Work out the finished part from the listing and answer in its coordinate system (mm). Coordinates: 2 decimals unless noted, no trailing zeros. Order: outer loops, then holes, each group sorted by start corner. A loop starts at its lowest first (then second) coordinate and runs counter-clockwise, first axis right, second up. Notation, with made-up numbers: (54, -4.75) -> (92, -4.75) arc R20 cw to (92, 29.25) -> close; hole circle Ø5 at (16.25, 82). An arc over 180 degrees is marked (long way). Use one line per item in the form item = value.
from build123d import *

# Parameters (mm, degrees)
F1_DEPTH      = 25.4
F1_DEPTH_BACK = 25.4


with BuildPart() as f1:
    # F0 (on Front) → F1 (new body, two sides)
    with BuildSketch(Plane.XZ) as f1_sk:
        Polygon((-66.331223, 8.359254), (-66.331223, 0), (85.438088, 0), (85.438088, 15.741451), (38.973667, 27.900366), (-1.845549, 27.900366), (-21.16954, 17.044192), align=None)
    extrude(amount=F1_DEPTH)
    extrude(f1_sk.sketch, amount=-F1_DEPTH_BACK)


solid = f1.part
(1) Each of these flat-tipped pins is pushed along its axis until it touches: P1, Ø1.5, axis at x = 66, y = -9.5, coming from the +Z side; P2, Ø4, axis at x = -46, y = 12, coming from the +Z side. Where does it stop, or does it pass through?
Data:
P1 = 21.02
P2 = 12.65
(2) Section C-C on x = -53 is taken. Write down the section's boundary in (y, z), plus the area to 3 significant figures.
Data:
outline = (-25.4, 0) -> (25.4, 0) -> (25.4, 10.92) -> (-25.4, 10.92) -> close
area = 555 mm²
(3) Section A-A on y = -11 is taken. Write down the section's boundary in (x, z), plus the area to 3 significant figures.
Data:
outline = (-66.33, 0) -> (85.44, 0) -> (85.44, 15.74) -> (38.97, 27.9) -> (-1.85, 27.9) -> (-21.17, 17.04) -> (-66.33, 8.36) -> close
area = 3,160 mm²
(4) Straight lines are drawn through the part: line 1 along Z through (x, y) = (-40.5, -15); line 2 along Z through (x, y) = (-50.5, -16). For each, find the intervals that lie inside material, in ascending order.
Data:
line_1 = 0 to 13.33
line_2 = 0 to 11.4
(5) Section B-B on x = -33.5 is taken. Write down the section's boundary in (y, z), plus the area to 3 significant figures.
Data:
outline = (-25.4, 0) -> (25.4, 0) -> (25.4, 14.67) -> (-25.4, 14.67) -> close
area = 745 mm²
